```python
from build123d import *

# Parameters (mm, degrees)
SKETCH1_W           = 40
SKETCH1_H           = 40
BOSS_EXTRUDE1_DEPTH = 5
FILLET1_R           = 2
SKETCH2_W           = 2
SKETCH2_H           = 36
BOSS_EXTRUDE2_DEPTH = 110
SKETCH3_W           = 40
SKETCH3_H           = 40
BOSS_EXTRUDE3_DEPTH = 3
FILLET2_R           = 2
SKETCH4_R           = 1.5
CUT_EXTRUDE1_DEPTH  = 10
SKETCH5_R           = 2.5
CUT_EXTRUDE2_DEPTH  = 127.368508888
SKETCH6_R           = 2.5
CUT_EXTRUDE4_DEPTH  = 131.858702575
SKETCH8_R           = 3.5
BOSS_EXTRUDE4_DEPTH = 114


with BuildPart() as part:
    # Sketch1 → Boss-Extrude1 (new body)
    with BuildSketch(Plane(origin=(0, 0, 0), x_dir=(1, 0, 0), z_dir=(0, 1, 0))):
        with Locations((20, -20)):
            Rectangle(SKETCH1_W, SKETCH1_H)
    extrude(amount=BOSS_EXTRUDE1_DEPTH)

    # Fillet1
    fillet1_edges = [part.edges().sort_by_distance(p)[0] for p in [
        (40, 2.5, 0),
        (40, 2.5, 40),
        (0, 2.5, 40),
        (0, 2.5, 0),
    ]]
    fillet(fillet1_edges, radius=FILLET1_R)

    # Sketch2 → Boss-Extrude2 (add)
    with BuildSketch(Plane.XZ):
        with Locations((1, 20)):
            Rectangle(SKETCH2_W, SKETCH2_H)
        with Locations((39, 20)):
            Rectangle(SKETCH2_W, SKETCH2_H)
    extrude(amount=BOSS_EXTRUDE2_DEPTH)

    # Sketch3 → Boss-Extrude3 (add)
    with BuildSketch(Plane.XZ.offset(110)):
        with Locations((20, 20)):
            Rectangle(SKETCH3_W, SKETCH3_H)
    extrude(amount=BOSS_EXTRUDE3_DEPTH)

    # Fillet2
    fillet2_edges = [part.edges().sort_by_distance(p)[0] for p in [
        (0, -111.5, 0),
        (40, -111.5, 0),
        (40, -111.5, 40),
        (0, -111.5, 40),
    ]]
    fillet(fillet2_edges, radius=FILLET2_R)

    # Sketch4 → Cut-Extrude1 (cut)
    with BuildSketch(Plane.XZ.offset(113)):
        with Locations(Location((4, 4, 0), (0, 0, 270))):
            Circle(SKETCH4_R)
        with Locations(Location((36, 4, 0), (0, 0, 270))):
            Circle(SKETCH4_R)
        with Locations(Location((4, 36, 0), (0, 0, 270))):
            Circle(SKETCH4_R)
        with Locations(Location((36, 36, 0), (0, 0, 270))):
            Circle(SKETCH4_R)
    extrude(amount=-CUT_EXTRUDE1_DEPTH, mode=Mode.SUBTRACT)

    # Sketch5 → Cut-Extrude2 (cut, through all)
    with BuildSketch(Plane(origin=(0, 0, 0), x_dir=(1, 0, 0), z_dir=(0, 1, 0))):
        with Locations(Location((20, -20, 0), (0, 0, 270))):
            Circle(SKETCH5_R)
    extrude(amount=CUT_EXTRUDE2_DEPTH, mode=Mode.SUBTRACT)

    # Sketch6 → Cut-Extrude4 (cut, through all)
    with BuildSketch(Plane.XZ.offset(113)):
        with Locations(Location((20, 20, 0), (0, 0, 90))):
            Circle(SKETCH6_R)
    extrude(amount=-CUT_EXTRUDE4_DEPTH, mode=Mode.SUBTRACT)

    # Sketch8 → Boss-Extrude4 (add)
    with BuildSketch(Plane(origin=(0, -110, 0), x_dir=(1, 0, 0), z_dir=(0, 1, 0))):
        with Locations(Location((9, -20, 0), (0, 0, 270))):
            Circle(SKETCH8_R)
        with Locations(Location((31, -20, 0), (0, 0, 270))):
            Circle(SKETCH8_R)
    extrude(amount=BOSS_EXTRUDE4_DEPTH)


solid = part.part
```
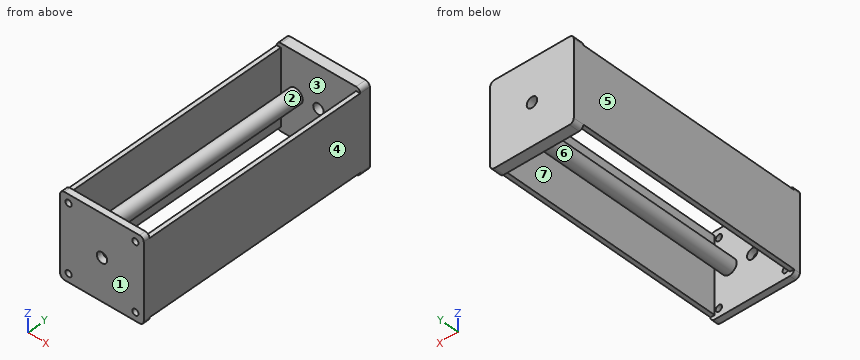
Here's how the part is built. I have some questions about the finished solid (model axes, mm). Face numbers are marked on the shaded views. A direction names the side the tool comes from. Give positions to 0.01 mm unless a question says otherwise; leave off trailing zeros. Loops run counter-clockwise (first coordinate to the right, second up) from the corner with the lowest first, then second, coordinate; pieces in that order, holes last. Notation, with made-up numbers: M 59.5,19.5 L 79.5,19.5 A17 cw 79.5,30.5 Z; hole C 11.25,74.5 d5. An arc over 180 degrees is marked long. Return JSON: item names as keys, results as strings.
Item 1: Imagine slicing it at A-A on z = 36. List the corners of the cut face in (x, y) for me.
A:
{"outline": "M 0,-113 L 2.5,-113 L 2.5,-110 L 2,-110 L 2,0 L 38,0 L 38,-110 L 37.5,-110 L 37.5,-113 L 40,-113 L 40,5 L 0,5 Z; M 5.5,-113 L 34.5,-113 L 34.5,-110 L 5.5,-110 Z"}
Item 2: Please list where these lines run through material, in increasing order: line 1 (X direction, y = -111.2, z = 4); line 2 (Y direction, x = 4.5, z = 37.5); line 3 (X direction, y = -87.5, z = 13.5).
A:
{"line 1": "x = 0 to 2.5, 5.5 to 34.5, 37.5 to 40", "line 2": "y = -113 to -110, 0 to 5", "line 3": "x = 0 to 2, 38 to 40"}
Item 3: Imagine slicing it at D-D on z = 20. List the corners of the cut face in (x, y) for me, then the cut area to 3 significant figures.
A:
{"outline": "M 0,-113 L 17.5,-113 L 17.5,-110 L 12.5,-110 L 12.5,0 L 17.5,0 L 17.5,5 L 0,5 Z; M 22.5,-113 L 40,-113 L 40,5 L 22.5,5 L 22.5,0 L 27.5,0 L 27.5,-110 L 22.5,-110 Z; hole M 2,-110 L 5.5,-110 L 5.5,0 L 2,0 Z; hole M 34.5,-110 L 38,-110 L 38,0 L 34.5,0 Z", "area": "2,260 mm^2"}
Item 4: Thinking about a two-plate mould opening in Y: for the marked faces 1, 2, 3 and 4, which applies, released by +Y, released by -Y, zero draft, split by the parting line, or undercut?
A:
{"face 1": "released by -Y", "face 2": "undercut", "face 3": "undercut", "face 4": "zero draft"}
Item 5: I'm going to push flat-ended pins straight in: pin 1 Ø10 at (x, y) = (16, -36) entering from -Z; pin 2 Ø2.5 at (x, z) = (4, 4) entering from -Y; pin 3 Ø2 at (x, y) = (11.5, -59.5) entering from +Z. Where does each tip first touch, or does it pass through?
A:
{"pin 1": "stops at z = 17.13", "pin 2": "stops at y = 0", "pin 3": "stops at z = 23.16"}
Item 6: On a 3-axis mill with a long thin cutter (end or side, diameter ignored), from which of +Z, -Z, +X, -X, +Y, -Y can I reach the whole of each face in a straight line? I mean the marked faces 5, 6 and 7. Say none if no direction works.
A:
{"face 5": "+Z, -Z, -X, +Y, -Y", "face 6": "none", "face 7": "+Z, -Z"}
Item 7: Imagine slicing it at B-B on x = 4. List the corners of the cut face in (y, z) for me.
A:
{"outline": "M -113,0 L -110,0 L -110,2.5 L -113,2.5 Z; M -113,5.5 L -110,5.5 L -110,34.5 L -113,34.5 Z; M -113,37.5 L -110,37.5 L -110,40 L -113,40 Z; M 0,0 L 5,0 L 5,40 L 0,40 Z"}
Item 8: Imagine slicing it at C-C on y = -24.5. List the corners of the cut face in (x, z) for me, then the cut area to 3 significant figures.
A:
{"outline": "M 0,2 L 2,2 L 2,38 L 0,38 Z; C 9,20 d7; C 31,20 d7; M 38,2 L 40,2 L 40,38 L 38,38 Z", "area": "221 mm^2"}
